Source: CAD feature listing. Evaluate the final solid. Frame: model axes, mm. A direction names the side the tool comes from. Round coordinates to 2 decimals unless told otherwise and drop trailing zeros. Return JSON: item names as keys, results as strings. Group by question number.
1) Contact query for flat-ended pins moving along their axis: P1, Ø1, axis at x = 56.5, z = -8.5, coming from the +Y side (3 decimals); P2, Ø2.5, axis at y = 7.5, z = -2.5, coming from the +X side. Output: stop coordinate, or through.
2) Ray query, line 1 (X direction, y = 8.25, z = -13.75); line 2 (X direction, y = 9.75, z = -6.25); line 3 (Y direction, x = 184, z = -5) (3 decimals). Return the intervals inside material, ascending. Write a range as from..to.
3) Access query for faces 1 (the flat face through (10.702, 17.336, -9.86)), 2 (the flat face through (3.35, 8, -3)), 3 (the flat face through (99, 10, 0)). Directions: +Z, -Z, +X, -X, +Y, -Y. A direction counts if a zero-diameter tool reaches every point of the face in a straight line with its end or side. Return the directions, or none.
4) Mould query, pull axis X, two halves, no side actions, for faces 4 (the flat face through (74.138, 17.289, -9.86)), 5 (the flat face through (1.28, 17.34, -9.86)), 6 (the flat face through (99, 10, -20)). Classes: pulls with the +X half, pulls with the -X half, needs draft (parallel to the pull), parting line crosses it, or undercut.
```python
from build123d import *

# Parameters (mm, degrees)
BLANKSKE_W          = 200
BLANKSKE_H          = 19
BLANK_DEPTH         = 20
TOOTHCUTSIM_DEPTH   = 202.893536301
TEETHCUTS_COUNT     = 43
TEETHCUTS_PITCH     = 4.712388975
SKETCH1_W           = 4.8
SKETCH1_H           = 19
BOSS_EXTRUDE1_DEPTH = 15
SKETCH2_W           = 15
SKETCH2_H           = 3.6
SKETCH2_W_2         = 3.4
SKETCH2_H_2         = 3.4
CUT_EXTRUDE1_DEPTH  = 4.8
SKETCH3_W           = 7
SKETCH3_H           = 7
CUT_EXTRUDE3_DEPTH  = 10
SKETCH4_W           = 3.3
SKETCH4_H           = 3.3
CUT_EXTRUDE4_DEPTH  = 25


with BuildPart() as part:
    # BlankSke → Blank (new body)
    with BuildSketch(Plane.XY):
        with Locations((100, 9.5)):
            Rectangle(BLANKSKE_W, BLANKSKE_H)
    extrude(amount=-BLANK_DEPTH)

    # TooCutSkeSim → ToothCutSim (cut, through all)
    with BuildSketch(Plane.XY):
        Polygon((0.654653055, 15.625), (-0.654653055, 15.625), (-1.892297439, 19.0254), (1.892297439, 19.0254), align=None)
    toothcutsim = extrude(amount=-TOOTHCUTSIM_DEPTH, mode=Mode.SUBTRACT)

    # TeethCuts: ToothCutSim ×43
    with Locations(*[(i * TEETHCUTS_PITCH, 0, 0) for i in range(1, TEETHCUTS_COUNT)]):
        add(toothcutsim, mode=Mode.SUBTRACT)

    # Sketch1 → Boss-Extrude1 (add)
    with BuildSketch(Plane(origin=(200, 0, 0), x_dir=(0, 0, -1), z_dir=(1, 0, 0))):
        with Locations((10, 9.5)):
            Rectangle(SKETCH1_W, SKETCH1_H)
    extrude(amount=BOSS_EXTRUDE1_DEPTH)

    # Sketch2 → Cut-Extrude1 (cut)
    with BuildSketch(Plane(origin=(0, 0, -12.4), x_dir=(-1, 0, 0), z_dir=(0, 0, -1))):
        with Locations((-207.5, 17.2)):
            Rectangle(SKETCH2_W, SKETCH2_H)
        with Locations((-207.5, 1.8)):
            Rectangle(SKETCH2_W, SKETCH2_H)
        with Locations((-207.5, 9.5)):
            Rectangle(SKETCH2_W_2, SKETCH2_H_2)
    extrude(amount=-CUT_EXTRUDE1_DEPTH, mode=Mode.SUBTRACT)

    # Sketch3 → Cut-Extrude3 (cut)
    with BuildSketch(Plane.ZY):
        with Locations((-10, 7.8125)):
            Rectangle(SKETCH3_W, SKETCH3_H)
    extrude(amount=-CUT_EXTRUDE3_DEPTH, mode=Mode.SUBTRACT)

    # Sketch4 → Cut-Extrude4 (cut)
    with BuildSketch(Plane(origin=(0, 0, -20), x_dir=(-1, 0, 0), z_dir=(0, 0, -1))):
        with Locations((-5, 7.8125)):
            Rectangle(SKETCH4_W, SKETCH4_H)
    extrude(amount=-CUT_EXTRUDE4_DEPTH, mode=Mode.SUBTRACT)


solid = part.part
```
Geometry check:
{
 "1": {"P1": "y = 15.625", "P2": "x = 200"},
 "2": {"line 1": "0..3.35, 6.65..200", "line 2": "0..200", "line 3": "0..15.625"},
 "3": {"face 1": "+Z, -Z, +Y", "face 2": "+Z, -Z", "face 3": "+Z, +X, -X, +Y, -Y"},
 "4": {"face 4": "undercut", "face 5": "pulls with the -X half", "face 6": "needs draft"}
}
